Drawing for the job (mm, zero at the part's lowest x, y, z). Round coordinates to 2 decimals unless told otherwise and drop trailing zeros. Loops run counter-clockwise (first coordinate to the right, second up) from the corner with the lowest first, then second, coordinate; pieces in that order, holes last. Notation, with made-up numbers: (71, 69) -> (107, 69) arc R25 cw to (107, 102) -> close; hole circle Ø1 at (-11, 71.25). An arc over 180 degrees is marked (long way). Put each result on its own line as item: value. Start each with the question number.
Item 1: Flat gauge pins, fed straight in: pin 1 Ø3 at (x, z) = (142.5, 8.5) entering from -Y; pin 2 Ø1.5 at (x, z) = (81, 4) entering from +Y; pin 3 Ø4 at (x, z) = (31, 1.5) entering from +Y. Where does each tip first touch, or does it go through?
Item 2: Cut at A-A, the plane y = 80. List the corners of the cut face in (x, z).
Item 3: Cut at C-C, the plane z = 7.25. List the corners of the cut face in (x, y).
Item 4: Drill centre lines: probe 1 along Y at (x, z) = (80, 2.05); probe 2 along Y at (x, z) = (92.5, 1); probe 3 along Y at (x, z) = (80, 5.75). Where is each one in solid material? Low to high. Write a range as [from, to].
Item 5: Cut at D-D, the plane y = 117.5. List the corners of the cut face in (x, z), plus the area to 3 significant figures.
Item 6: Pull direction Y, two halves, no side cores. Call the marked faces 1, 2 and 3: +Y half, -Y half, draft (parallel to the pull), parting line (faces both ways), or undercut.
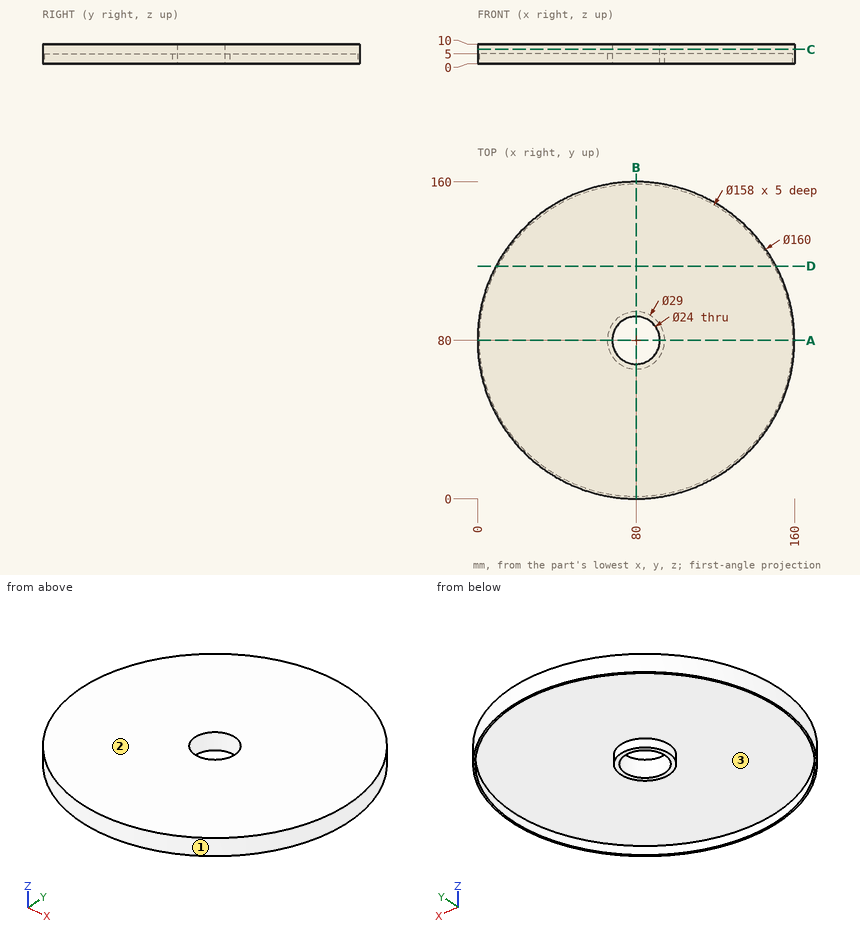
Reply:
1. pin 1: stops at y = 28.24
1. pin 2: stops at y = 160
1. pin 3: stops at y = 144.74
2. outline: (0, 0) -> (1, 0) -> (1, 5) -> (65.5, 5) -> (65.5, 0) -> (68, 0) -> (68, 10) -> (0, 10) -> close; (92, 0) -> (94.5, 0) -> (94.5, 5) -> (159, 5) -> (159, 0) -> (160, 0) -> (160, 10) -> (92, 10) -> close
3. outline: circle Ø160 at (80, 80); hole circle Ø24 at (80, 80)
4. probe 1: y = [0, 1], [65.5, 68], [92, 94.5], [159, 160]
4. probe 2: y = [0.98, 2], [72.65, 87.35], [158, 159.02]
4. probe 3: y = [0, 68], [92, 160]
5. outline: (9.33, 0) -> (10.47, 0) -> (10.47, 5) -> (149.53, 5) -> (149.53, 0) -> (150.67, 0) -> (150.67, 10) -> (9.33, 10) -> close
5. area: 718 mm^2
6. face 1: parting line
6. face 2: draft
6. face 3: undercut
